Build history of the part. All positions in model axes, mm. A direction names the side the tool comes from. Coordinates: 2 decimals unless noted, no trailing zeros. Order: outer loops, then holes, each group sorted by start corner. A loop starts at its lowest first (then second) coordinate and runs counter-clockwise, first axis right, second up. Notation, with made-up numbers: (76.5, 50.25) - (127.5, 50.25) arc R28 cw to (127.5, 88.25) - close; hole circle Ø3 at (89, -27). An arc over 180 degrees is marked (long way). Write each question's results on one line, items separated by ' | '.
from build123d import *

# Parameters (mm, degrees)
BOSS_EXTRUDE1_DEPTH = 1.5625
SKETCH2_W           = 15
SKETCH2_H           = 22.4625
CUT_EXTRUDE1_DEPTH  = 4.125
FILLET1_R           = 10
FILLET2_R           = 2


with BuildPart() as part:
    # Sketch1 → Boss-Extrude1 (new body, symmetric)
    with BuildSketch(Plane(origin=(0, 0, 0), x_dir=(1, 0, 0), z_dir=(0, 1, 0))):
        Polygon((0, 36), (35, 36), (35, 26.5), (28.5, 26.5), (28.5, 28.5), (26, 28.5), (26, 26.5), (24, 26.5), (24, 23.5), (26, 23.5), (26, 21.5), (28.5, 21.5), (28.5, 23.5), (35, 23.5), (35, 0), (0, 0), align=None)
    boss_extrude1 = extrude(amount=BOSS_EXTRUDE1_DEPTH, both=True)

    # Mirror1: Boss-Extrude1 across plane
    add(boss_extrude1.mirror(Plane(origin=(0, 0, 0), x_dir=(0, 0, 1), z_dir=(1, 0, 0))))

    # Sketch2 → Cut-Extrude1 (cut, through all)
    with BuildSketch(Plane.XZ.offset(1.5625)):
        with Locations((0, -11.23125)):
            Rectangle(SKETCH2_W, SKETCH2_H)
    extrude(amount=-CUT_EXTRUDE1_DEPTH, mode=Mode.SUBTRACT)

    # Fillet1
    fillet1_edges = [part.edges().sort_by_distance(p)[0] for p in [
        (-7.5, 0, 0),
        (7.5, 0, 0),
    ]]
    fillet(fillet1_edges, radius=FILLET1_R)

    # Fillet2
    fillet2_edges = [part.edges().sort_by_distance(p)[0] for p in [
        (-7.5, 0, -22.4625),
        (7.5, 0, -22.4625),
    ]]
    fillet(fillet2_edges, radius=FILLET2_R)


solid = part.part
1. Tool access for faces 5 (the face through (10.51, 0.02, -2.85)), 6 (the face through (-24, 0, -25)), 7 (the face through (28.5, 0, -22)): list every direction of +Z, -Z, +X, -X, +Y, -Y with a clear straight run to the whole face (end or side of a thin tool).
Solved:
face 5: +Z, +Y, -Y | face 6: -X, +Y, -Y | face 7: +Y, -Y
2. Two-plate mould, pull along Z, no slides. Class faces 1 (the face through (6.93, 0.02, -21.86)), 2 (the face through (26, 0, -23)), 3 (the face through (-35, 0, -12)), 4 (the face through (0, 0, -36)): +Z half, -Z half, draft (parallel to the pull), parting line (faces both ways), or undercut.
Solved:
face 1: +Z half | face 2: undercut | face 3: draft | face 4: -Z half
3. Band-saw the part on A-A on z = -11.5. Give the cut face in (x, y).
Solved:
outline: (-35, -1.56) - (-7.5, -1.56) - (-7.5, 1.56) - (-35, 1.56) - close; (7.5, -1.56) - (35, -1.56) - (35, 1.56) - (7.5, 1.56) - close
4. Probe line 1 (X direction, y = 0.5, z = -20); line 2 (Z direction, x = 32, y = 0.3); line 3 (X direction, y = 0.45, z = -26). List the from-to ranges inside material, lowest first.
Solved:
line 1: x = -35 to -7.5, 7.5 to 35 | line 2: z = -36 to -26.5, -23.5 to 0 | line 3: x = -24 to 24
5. Band-saw the part on B-B on z = -27.5. Give the cut face in (x, y).
Solved:
outline: (-35, -1.56) - (-28.5, -1.56) - (-28.5, 1.56) - (-35, 1.56) - close; (-26, -1.56) - (26, -1.56) - (26, 1.56) - (-26, 1.56) - close; (28.5, -1.56) - (35, -1.56) - (35, 1.56) - (28.5, 1.56) - close
6. Drop a flat-ended pin along its axis: pin 1 Ø2 at (x, z) = (5, -18.5) entering from +Y. Give the stop position or say it passes through.
Solved:
pin 1: passes through
7. Band-saw the part on C-C on z = -4. Give the cut face in (x, y), then the cut area to 3 significant figures.
Solved:
outline: (-35, -1.56) - (-9.5, -1.56) - (-9.5, 1.56) - (-35, 1.56) - close; (9.5, -1.56) - (35, -1.56) - (35, 1.56) - (9.5, 1.56) - close | area: 159 mm2
8. Band-saw the part on D-D on x = 3. Give the cut face in (y, z).
Solved:
outline: (-1.56, -36) - (1.56, -36) - (1.56, -22.46) - (-1.56, -22.46) - close
